The model under review builds one solid part; all positions refer to its coordinate system, in mm. Coordinates: 2 decimals unless noted, no trailing zeros. Write each loop counter-clockwise with the first axis right and the second up, starting at its lowest first coordinate (ties: lowest second). Pieces come first, ordered by that corner, then holes. Notation, with made-up numbers: (34.5, 41) - (73.5, 41) arc R14 cw to (73.5, 66) - close; hole circle Ø11 at (-5, -24.75). An arc over 180 degrees is marked (long way). Put each result on its own line as item: value. Start each with the question number.
Item 1: Consider section A-A on y = 0. Give the boundary of the cut face in (x, z).
Item 2: Mouldability with a two-part tool opening along Y and no side actions: class faces 1 (the face through (0, 0, 1)), 2 (the face through (1.052, -4.737, -2.668)), 3 (the face through (-4, -4, 0)) as pulls with the +Y half, pulls with the -Y half, needs draft (parallel to the pull), parting line crosses it, or undercut.
Item 3: Consider section B-B on x = 0. Give the boundary of the cut face in (y, z), then the cut area to 3 significant figures.
Item 4: Consider section C-C on z = 0.5. Give the boundary of the cut face in (x, y).
Item 5: For pin 1 (0.9 mm diameter, centred on y = -2, z = 1.5, fed in from +X); pin 2 (1.5 mm diameter, centred on x = -5, y = -7.5, fed in from -Z); pin 3 (3 mm diameter, centred on y = -7.5, z = 1, fed in from -X), all flat-tipped, find the tip position at first contact; note any pin that passes through.
Item 6: To check wall thickness, follow L1, parallel to Z at x = 5.5, y = 4.5; L2, parallel to X at y = 6, z = 1.25; L3, parallel to X at y = 3, z = 1.25. State the ranges of each line that lie inside material, in increasing order. Write a range as [from, to].
Item 7: Consider section D-D on z = -2.75. Give the boundary of the cut face in (x, y), then the cut area to 3 significant figures.
```python
from build123d import *

# Parameters (mm, degrees)
SKETCH1_R           = 9.6
BOSS_EXTRUDE2_DEPTH = 2
CHAMFER1_SIZE       = 1
FILLET1_R           = 0.3
SKETCH2_W           = 0.926275652
SKETCH2_H           = 12.346112468
CUT_EXTRUDE1_DEPTH  = 1
FILLET2_R           = 0.2
SKETCH5_R           = 4.852441015
BOSS_EXTRUDE3_DEPTH = 5
FILLET3_R           = 0.4


with BuildPart() as part:
    # Sketch1 → Boss-Extrude2 (new body)
    with BuildSketch(Plane.XY):
        Circle(SKETCH1_R)
    extrude(amount=BOSS_EXTRUDE2_DEPTH)

    # Chamfer1
    chamfer1_edges = [part.edges().sort_by_distance(p)[0] for p in [
        (-9.6, 0, 0),
    ]]
    chamfer(chamfer1_edges, length=CHAMFER1_SIZE)

    # Fillet1
    fillet1_edges = [part.edges().sort_by_distance(p)[0] for p in [
        (-9.6, 0, 2),
    ]]
    fillet(fillet1_edges, radius=FILLET1_R)

    # Sketch2 → Cut-Extrude1 (cut)
    with BuildSketch(Plane.XY.offset(2)):
        Rectangle(SKETCH2_W, SKETCH2_H)
    extrude(amount=-CUT_EXTRUDE1_DEPTH, mode=Mode.SUBTRACT)

    # Fillet2
    fillet2_edges = [part.edges().sort_by_distance(p)[0] for p in [
        (0.463137826, 6.173056234, 1.5),
        (0, -6.173056234, 1),
        (0.463137826, -6.173056234, 1.5),
        (-0.463137826, -6.173056234, 1.5),
        (-0.463137826, 6.173056234, 1.5),
        (0.463137826, 0, 2),
        (0, 6.173056234, 2),
        (-0.463137826, 0, 2),
        (0, -6.173056234, 2),
    ]]
    fillet(fillet2_edges, radius=FILLET2_R)

    # Sketch5 → Boss-Extrude3 (add)
    with BuildSketch(Plane(origin=(0, 0, 0), x_dir=(-1, 0, 0), z_dir=(0, 0, -1))):
        Circle(SKETCH5_R)
    extrude(amount=BOSS_EXTRUDE3_DEPTH)

    # Fillet3
    fillet3_edges = [part.edges().sort_by_distance(p)[0] for p in [
        (4.852441015, 0, 0),
        (-8.6, 0, 0),
    ]]
    fillet(fillet3_edges, radius=FILLET3_R)


solid = part.part
```
Report:
1. outline: (-9.6, 1) - (-8.72, 0.12) arc R0.4 ccw to (-8.43, 0) - (-5.25, 0) arc R0.4 cw to (-4.85, -0.4) - (-4.85, -5) - (4.85, -5) - (4.85, -0.4) arc R0.4 cw to (5.25, 0) - (8.43, 0) arc R0.4 ccw to (8.72, 0.12) - (9.6, 1) - (9.6, 1.7) arc R0.3 ccw to (9.3, 2) - (0.66, 2) arc R0.2 ccw to (0.46, 1.8) - (0.46, 1) - (-0.46, 1) - (-0.46, 1.8) arc R0.2 ccw to (-0.66, 2) - (-9.3, 2) arc R0.3 ccw to (-9.6, 1.7) - close
2. face 1: undercut
2. face 2: parting line crosses it
2. face 3: needs draft
3. outline: (-9.6, 1) - (-8.72, 0.12) arc R0.4 ccw to (-8.43, 0) - (-5.25, 0) arc R0.4 cw to (-4.85, -0.4) - (-4.85, -5) - (4.85, -5) - (4.85, -0.4) arc R0.4 cw to (5.25, 0) - (8.43, 0) arc R0.4 ccw to (8.72, 0.12) - (9.6, 1) - (9.6, 1.7) arc R0.3 ccw to (9.3, 2) - (6.37, 2) arc R0.2 ccw to (6.17, 1.8) - (6.17, 1) - (-5.97, 1) arc R0.2 cw to (-6.17, 1.2) - (-6.17, 1.8) arc R0.2 ccw to (-6.37, 2) - (-9.3, 2) arc R0.3 ccw to (-9.6, 1.7) - close
3. area: 73.6 mm²
4. outline: circle Ø18.2 at (0, 0)
5. pin 1: x = 9.47
5. pin 2: z = 0
5. pin 3: x = -7.49
6. L1: [0, 2]
6. L2: [-7.49, -0.46], [0.46, 7.49]
6. L3: [-9.12, -0.46], [0.46, 9.12]
7. outline: circle Ø9.7 at (0, 0)
7. area: 74.0 mm²
